```python
from build123d import *

# Parameters (mm, degrees)
BOSS_EXTRUDE1_DEPTH = 50
SKETCH2_R           = 5
CUT_EXTRUDE1_DEPTH  = 25
SKETCH3_R           = 7.5
CUT_EXTRUDE2_DEPTH  = 25


with BuildPart() as part:
    # Sketch1 → Boss-Extrude1 (new, symmetric)
    with BuildSketch(Plane.XY):
        Polygon((27.5, 45), (-27.5, 45), (-57.5, 5), (-85, 5), (-85, 0), (-55, 0), (-25, 40), (25, 40), (55, 0), (85, 0), (85, 5), (57.5, 5), align=None)
    extrude(amount=BOSS_EXTRUDE1_DEPTH, both=True)

    # Sketch2 → Cut-Extrude1 (cut, symmetric)
    with BuildSketch(Plane(origin=(0, 5, 0), x_dir=(1, 0, 0), z_dir=(0, 1, 0))):
        with Locations(Location((-71.25, -40, 0), (0, 0, 180))):
            Circle(SKETCH2_R)
        with Locations(Location((-71.25, -20, 0), (0, 0, 180))):
            Circle(SKETCH2_R)
        with Locations(Location((-71.25, 0, 0), (0, 0, 180))):
            Circle(SKETCH2_R)
        with Locations(Location((-71.25, 20, 0), (0, 0, 180))):
            Circle(SKETCH2_R)
        with Locations(Location((-71.25, 40, 0), (0, 0, 180))):
            Circle(SKETCH2_R)
    cut_extrude1 = extrude(amount=CUT_EXTRUDE1_DEPTH, both=True, mode=Mode.SUBTRACT)

    # Mirror1: Cut-Extrude1 across plane
    add(cut_extrude1.mirror(Plane(origin=(0, 0, 0), x_dir=(0, 0, 1), z_dir=(1, 0, 0))), mode=Mode.SUBTRACT)

    # Sketch3 → Cut-Extrude2 (cut, symmetric)
    with BuildSketch(Plane(origin=(0, 45, 0), x_dir=(1, 0, 0), z_dir=(0, 1, 0))):
        with Locations(Location((0, -30, 0), (0, 0, 270))):
            Circle(SKETCH3_R)
        with Locations(Location((0, 30, 0), (0, 0, 270))):
            Circle(SKETCH3_R)
    extrude(amount=CUT_EXTRUDE2_DEPTH, both=True, mode=Mode.SUBTRACT)


solid = part.part
```
Can you work these out from the model? Positions are in its coordinate system, mm. A direction names the side the tool comes from. Give positions to 0.01 mm unless a question says otherwise; leave off trailing zeros. Loops run counter-clockwise (first coordinate to the right, second up) from the corner with the lowest first, then second, coordinate; pieces in that order, holes last. Notation, with made-up numbers: M 44.25,54.5 L 86.25,54.5 A27 ccw 86.25,79.5 Z; hole C 53.25,42 d3. An arc over 180 degrees is marked long. One line per question, with ' | ' between items. Start each with the question number.
Q1. For faces 1 (the flat face through (65, 5, 1)), 2 (the flat face through (-40, 20, 1)), 3 (the flat face through (-64, 0, 1)), 4 (the flat face through (-77, 5, 1)), which set-ups out of +Z, -Z, +X, -X, +Y, -Y let a thin tool reach every point of the face, with its end or its side?
Q2. For pin 1 Ø10 at (y, z) = (25.5, 23.5) entering from -X (3 decimals); pin 2 Ø16 at (x, z) = (-71.25, -40) entering from -Y; pin 3 Ø6 at (x, z) = (71.25, -40) entering from -Y; pin 4 Ø11.5 at (x, z) = (71.25, 0) entering from +Y, each with a flat end and sliding along its axis, tell me the tip position at first contact or that it passes through.
Q3. If we mould it in two halves opening along Z, with no side actions, what happens to faces 5 (the flat face through (-42.29, 25.28, 0.7)), 6 (the cylindrical face through (-76.02, 2.54, -38.5)), 7 (the flat face through (0, 41, -50))? For each: +Z half, -Z half, draft (parallel to the pull), parting line (faces both ways), or undercut.
Q4. If we section it at C-C (y = 21.5): Please give me the cut outline in (x, z) (3 decimals).
Q5. If we section it at A-A (x = 71.25): Please give me the cut outline in (y, z), plus the area to 3 significant figures.
Q6. If we section it at D-D (z = -40): Please give me the cut outline in (x, y).
Q7. If we section it at B-B (z = 30): Please give me the cut outline in (x, y), plus the area to 3 significant figures.
Q8. If I drill on line 1 (Z direction, x = -71, y = 3); line 2 (Y direction, x = -76, z = -22.5); line 3 (Y direction, x = 12.5, z = -19), over which ranges is the centre line in solid material (lowest first)? Write a range as from..to.
Computed:
1) face 1: +Z, -Z, +X, +Y | face 2: +Z, -Z, -Y | face 3: +Z, -Z, +X, -X, -Y | face 4: +Z, -Z, -X, +Y
2) pin 1: stops at x = -45.875 | pin 2: stops at y = 0 | pin 3: passes through | pin 4: stops at y = 5
3) face 5: draft | face 6: undercut | face 7: -Z half
4) outline: M -45.125,-50 L -38.875,-50 L -38.875,50 L -45.125,50 Z; M 38.875,-50 L 45.125,-50 L 45.125,50 L 38.875,50 Z
5) outline: M 0,-50 L 5,-50 L 5,-45 L 0,-45 Z; M 0,-35 L 5,-35 L 5,-25 L 0,-25 Z; M 0,-15 L 5,-15 L 5,-5 L 0,-5 Z; M 0,5 L 5,5 L 5,15 L 0,15 Z; M 0,25 L 5,25 L 5,35 L 0,35 Z; M 0,45 L 5,45 L 5,50 L 0,50 Z | area: 250 mm²
6) outline: M -85,0 L -76.25,0 L -76.25,5 L -85,5 Z; M -66.25,0 L -55,0 L -25,40 L 25,40 L 55,0 L 66.25,0 L 66.25,5 L 57.5,5 L 27.5,45 L -27.5,45 L -57.5,5 L -66.25,5 Z; M 76.25,0 L 85,0 L 85,5 L 76.25,5 Z
7) outline: M -85,0 L -55,0 L -25,40 L -7.5,40 L -7.5,45 L -27.5,45 L -57.5,5 L -85,5 Z; M 7.5,40 L 25,40 L 55,0 L 85,0 L 85,5 L 57.5,5 L 27.5,45 L 7.5,45 Z | area: 975 mm²
8) line 1: z = -50..-44.99, -35.01..-24.99, -15.01..-4.99, 4.99..15.01, 24.99..35.01, 44.99..50 | line 2: y = 0..5 | line 3: y = 40..45
